Design review of the part built by this model. Coordinates are the model's own, in mm. A direction names the side the tool comes from. Coordinates: 2 decimals unless noted, no trailing zeros. Order: outer loops, then holes, each group sorted by start corner. A loop starts at its lowest first (then second) coordinate and runs counter-clockwise, first axis right, second up. Notation, with made-up numbers: (73, -16.5) -> (128, -16.5) arc R33 ccw to (128, 14.5) -> close; hole circle Ø7 at (69, -27.5). An arc over 180 degrees is marked (long way). Use a Markdown table: item, result. Add a question column.
Q1. Wall thickness on probe 1 along Z at (x, y) = (-5, 0.45); probe 2 along Y at (x, z) = (-10, 18.25); probe 3 along X at (y, z) = (5, 1.5): over which ranges is each line inside the solid? List them lowest first.
Q2. Add section D-D (y = 5.25). State the section outline as (x, z) points.
Q3. The part is to be moulded in two halves that separate along Z. For faces 1 (the face through (-8.8, 11.2, 0)), 2 (the face through (-11, 1, 12)), 3 (the face through (-5.33, 0.49, 17.38)), say which applies: pulls with the +Z half, pulls with the -Z half, needs draft (parallel to the pull), parting line crosses it, or undercut.
Q4. Add section C-C (z = 8.25). State the section outline as (x, y) points.
Q5. Add section B-B (x = -21). State the section outline as (y, z) points.
Q6. Insertion check: pin 1 (3 mm diameter, centred on y = 5.5, z = 9, fed in from +X); pin 2 (7.5 mm diameter, centred on x = -9.5, z = 8, fed in from +Y); pin 3 (1 mm diameter, centred on y = 12, z = 16, fed in from -X). Each pin has a flat end and moves straight along its axis. Give the tip position at first contact, or say it passes through.
Q7. Machinability: for faces 4 (the face through (-4, 12, 12)), 5 (the face through (-3, 11, 12)), 6 (the face through (-6.19, 0.49, 2.99)), 7 (the face through (0, 0.5, 12.3)), which of the approach directions +Z, -Z, +X, -X, +Y, -Y give a long, thin tool a straight path to every point of the face, cutting with its end or side? Answer none if there is none.
Q8. Add section A-A (x = -5). State the section outline as (y, z) points.
from build123d import *

# Parameters (mm, degrees)
EXTRUS_O_FINA1_DEPTH  = 25
ESBO_O2_R             = 1.5
CORTE_EXTRUS_O1_DEPTH = 5


with BuildPart() as part:
    # Esboço1 → Extrusão-Fina1 (new body)
    with BuildSketch(Plane.XY):
        with BuildLine():
            Line((0, 0), (-22, 0))
            ThreePointArc((-22, 0), (-24.121320344, 0.878679656), (-25, 3))
            Line((-25, 3), (-25, 9))
            ThreePointArc((-25, 9), (-24.121320344, 11.121320344), (-22, 12))
            Line((-22, 12), (-10, 12))
            Line((-10, 12), (13.964550925, 12))
            Line((13.964550925, 12), (15.645056047, 14.73834825))
            Line((15.645056047, 14.73834825), (16.497357261, 14.215296971))
            Line((16.497357261, 14.215296971), (14.524152053, 11))
            Line((14.524152053, 11), (-10, 11))
            Line((-10, 11), (-22, 11))
            ThreePointArc((-22, 11), (-23.414213562, 10.414213562), (-24, 9))
            Line((-24, 9), (-24, 3))
            ThreePointArc((-24, 3), (-23.414213562, 1.585786438), (-22, 1))
            Line((-22, 1), (0, 1))
            Line((0, 1), (0, 0))
        make_face()
    extrude(amount=EXTRUS_O_FINA1_DEPTH)

    # Esboço2 → Corte-extrusão1 (cut)
    with BuildSketch(Plane.XZ):
        with Locations((-5, 18.842376972)):
            Circle(ESBO_O2_R)
        with Locations((-5, 3.904607357)):
            Circle(ESBO_O2_R)
    extrude(amount=-CORTE_EXTRUS_O1_DEPTH, mode=Mode.SUBTRACT)


solid = part.part
Established:
| question | item | result |
|---|---|---|
| 1 | probe 1 | 0 to 2.4, 5.4 to 17.34, 20.34 to 25 |
| 1 | probe 2 | 0 to 1, 11 to 12 |
| 1 | probe 3 | -25 to -24 |
| 2 | outline | (-25, 0) -> (-24, 0) -> (-24, 25) -> (-25, 25) -> close |
| 3 | face 1 | pulls with the -Z half |
| 3 | face 2 | needs draft |
| 3 | face 3 | undercut |
| 4 | outline | (-25, 3) arc R3 ccw to (-22, 0) -> (0, 0) -> (0, 1) -> (-22, 1) arc R2 cw to (-24, 3) -> (-24, 9) arc R2 cw to (-22, 11) -> (14.52, 11) -> (16.5, 14.22) -> (15.65, 14.74) -> (13.96, 12) -> (-22, 12) arc R3 ccw to (-25, 9) -> close |
| 5 | outline | (0, 0) -> (1, 0) -> (1, 25) -> (0, 25) -> close; (11, 0) -> (12, 0) -> (12, 25) -> (11, 25) -> close |
| 6 | pin 1 | x = -24 |
| 6 | pin 2 | y = 12 |
| 6 | pin 3 | x = -23.66 |
| 7 | face 4 | +Z, -Z, -X, +Y |
| 7 | face 5 | +Z, -Z, +X |
| 7 | face 6 | -Y |
| 7 | face 7 | +Z, -Z, +X, -Y |
| 8 | outline | (0, 0) -> (1, 0) -> (1, 2.4) -> (0, 2.4) -> close; (0, 5.4) -> (1, 5.4) -> (1, 17.34) -> (0, 17.34) -> close; (0, 20.34) -> (1, 20.34) -> (1, 25) -> (0, 25) -> close; (11, 0) -> (12, 0) -> (12, 25) -> (11, 25) -> close |
